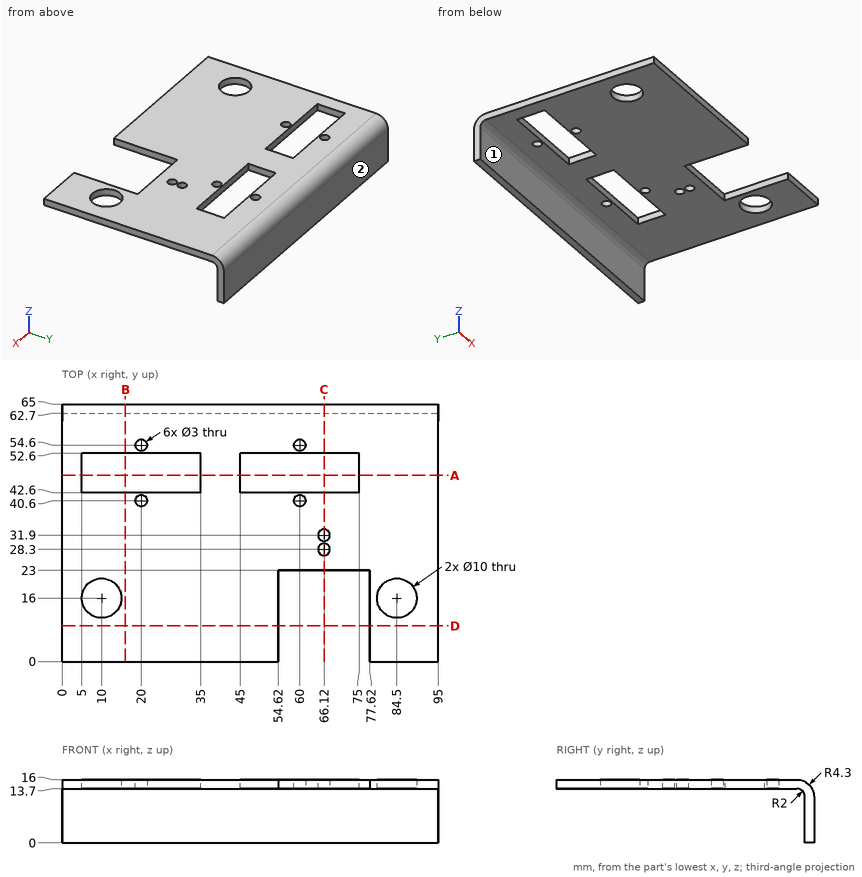
Answer from the drawing. Dimensions are ordinates in mm from the lowest x, y and z of the part. A direction names the side the tool comes from. Round coordinates to 2 decimals unless told otherwise and drop trailing zeros. Loops run counter-clockwise (first coordinate to the right, second up) from the corner with the lowest first, then second, coordinate; pieces in that order, holes last.
1) For the marked faces 1 and 2, determine the directions among +Z, -Z, +X, -X, +Y, -Y from which every point of the face is accessible in a straight line to the end or side of a thin tool.
Outcome:
face 1: -Z, +X, -X, -Y
face 2: +Z, -Z, +X, -X, +Y
2) A cutting plane is placed at A-A on y = 47. Determine the outline of the cut face in (x, z).
Outcome:
outline: (0, 13.7) - (5, 13.7) - (5, 16) - (0, 16) - close; (35, 13.7) - (45, 13.7) - (45, 16) - (35, 16) - close; (75, 13.7) - (95, 13.7) - (95, 16) - (75, 16) - close
3) Given P1, Ø18, axis at x = 40, y = 26.5, coming from the -Z side; P2, Ø2.5, axis at x = 58.5, z = 14.5, coming from the +Y side; P3, Ø1.2, axis at x = 66.5, z = 14.5, coming from the -Y side, each flat-ended and moving along its own axis, determine where each tip first touches the part or whether it passes through.
Outcome:
P1: stops at z = 13.7
P2: stops at y = 64.71
P3: stops at y = 23
4) A cutting plane is placed at C-C on x = 66.12. Determine the outline of the cut face in (y, z), plus the area to 3 significant figures.
Outcome:
outline: (23, 13.7) - (26.8, 13.7) - (26.8, 16) - (23, 16) - close; (29.8, 13.7) - (30.4, 13.7) - (30.4, 16) - (29.8, 16) - close; (33.4, 13.7) - (42.6, 13.7) - (42.6, 16) - (33.4, 16) - close; (52.6, 13.7) - (60.7, 13.7) arc R2 cw to (62.7, 11.7) - (62.7, 0) - (65, 0) - (65, 11.7) arc R4.3 ccw to (60.7, 16) - (52.6, 16) - close
area: 88.2 mm2
5) A cutting plane is placed at B-B on x = 16. Determine the outline of the cut face in (y, z).
Outcome:
outline: (0, 13.7) - (42.6, 13.7) - (42.6, 16) - (0, 16) - close; (52.6, 13.7) - (60.7, 13.7) arc R2 cw to (62.7, 11.7) - (62.7, 0) - (65, 0) - (65, 11.7) arc R4.3 ccw to (60.7, 16) - (52.6, 16) - close
6) Consider line 1 (X direction, y = 43, z = 13.75); line 2 (Y direction, x = 60, z = 15.05); line 3 (Z direction, x = 8.5, y = 55.5). Determine where each line is inside the solid, lowest interval first.
Outcome:
line 1: x = 0 to 5, 35 to 45, 75 to 95
line 2: y = 23 to 39.1, 42.1 to 42.6, 52.6 to 53.1, 56.1 to 63.4
line 3: z = 13.7 to 16
7) A cutting plane is placed at D-D on y = 9. Determine the outline of the cut face in (x, z).
Outcome:
outline: (0, 13.7) - (54.62, 13.7) - (54.62, 16) - (0, 16) - close; (77.62, 13.7) - (95, 13.7) - (95, 16) - (77.62, 16) - close
